Read the model definition and answer for the solid it produces. Units are mm, in the model's axes. Round coordinates to 2 decimals unless told otherwise and drop trailing zeros. Write each loop counter-clockwise with the first axis right and the second up, starting at its lowest first coordinate (ties: lowest second). Pieces come first, ordered by that corner, then holes. Notation, with made-up numbers: (73, 28.25) - (108, 28.25) arc R34 ccw to (108, 66.25) - close; hole circle Ø8 at (-34, 83). An arc over 180 degrees is marked (long way). Use one line per item in the form item = value. Start each with the question number.
1) Each of these flat-tipped pins is pushed along its axis until it touches: pin 1 (1 mm diameter, centred on x = -44, z = 2, fed in from -Y); pin 2 (1.6 mm diameter, centred on x = -27.5, z = 1.5, fed in from -Y); pin 3 (1 mm diameter, centred on y = -2, z = 1, fed in from -X) (3 decimals). Where does it stop, or does it pass through?
2) The part is cut by section C-C, the plane x = -27.5. Give the vertices of the cut face in (y, z) (3 decimals).
3) The part is cut by section B-B, the plane z = 1.35. Give the vertices of the cut face in (x, y) (3 decimals), plus the area to 3 significant figures.
4) Consider line 1 along X through (y, z) = (3.5, 0.85) (3 decimals); line 2 along Y through (x, z) = (-24.5, 2.75); line 3 along Y through (x, z) = (0.5, 2.4). Determine where each line is inside the solid, lowest interval first. Write a range as from..to.
5) The part is cut by section D-D, the plane y = 52.5. Give the vertices of the cut face in (x, z) (3 decimals), plus the area to 3 significant figures.
6) The part is cut by section A-A, the plane y = 3.5. Give the vertices of the cut face in (x, z) (3 decimals), plus the area to 3 significant figures.
from build123d import *

# Parameters (mm, degrees)
BOSS_EXTRUDE1_DEPTH = 3.175
KERF_DEPTH          = 3.175


with BuildPart() as part:
    # Sketch1 → Boss-Extrude1 (new body)
    with BuildSketch(Plane.XY):
        Polygon((0, 0), (-6.35, 0), (-6.35, -3.81), (-19.05, -3.81), (-19.05, 0), (-25.4, 0), (-25.4, 18.4658), (-28.575, 18.4658), (-28.575, 0), (-28.575, -3.81), (-41.275, -3.81), (-41.275, 0), (-47.625, 0), (-47.625, 6.35), (-25.4, 63.5), (0, 63.5), (0, 57.15), (3.048, 57.15), (3.048, 38.1), (0, 38.1), (0, 31.75), (3.048, 31.75), (3.048, 12.7), (0, 12.7), align=None)
    extrude(amount=BOSS_EXTRUDE1_DEPTH)

    # Sketch2 → kerf (add, through all)
    with BuildSketch(Plane.XY.offset(3.175)):
        Polygon((-25.4, 0), (-19.05, 0), (-19.05, -3.81), (-6.35, -3.81), (-6.35, 0), (0, 0), (0, 12.7), (3.048, 12.7), (3.048, 31.75), (0, 31.75), (0, 38.1), (3.048, 38.1), (3.048, 57.15), (0, 57.15), (0, 63.5), (-25.4, 63.5), (-47.625, 6.35), (-47.625, 0), (-41.275, 0), (-41.275, -3.81), (-28.575, -3.81), (-28.575, 18.4658), (-25.4, 18.4658), align=None)
    extrude(amount=-KERF_DEPTH)


solid = part.part
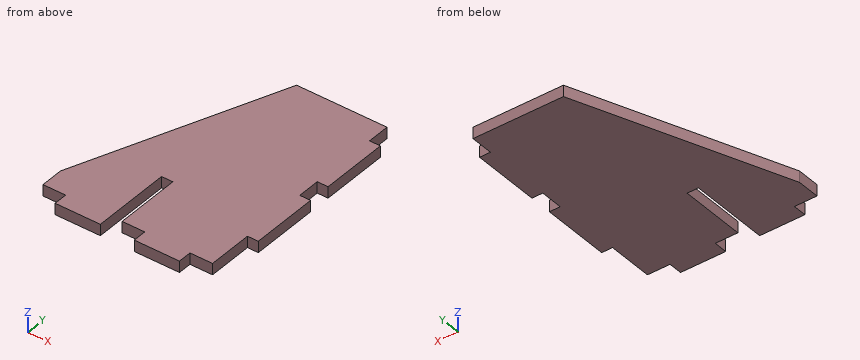
Geometry results:
q1.pin_1 = 0
q1.pin_2 = 18.47
q1.pin_3 = -41.275
q2.outline = (18.466, 0) - (58.1, 0) - (58.1, 3.175) - (18.466, 3.175) - close
q3.outline = (-47.625, 0) - (-41.275, 0) - (-41.275, -3.81) - (-28.575, -3.81) - (-28.575, 18.466) - (-25.4, 18.466) - (-25.4, 0) - (-19.05, 0) - (-19.05, -3.81) - (-6.35, -3.81) - (-6.35, 0) - (0, 0) - (0, 12.7) - (3.048, 12.7) - (3.048, 31.75) - (0, 31.75) - (0, 38.1) - (3.048, 38.1) - (3.048, 57.15) - (0, 57.15) - (0, 63.5) - (-25.4, 63.5) - (-47.625, 6.35) - close
q3.area = 2,540 mm2
q4.line_1 = -47.625..-28.575, -25.4..0
q4.line_2 = 0..63.5
q4.line_3 = 12.7..31.75, 38.1..57.15
q5.outline = (-29.678, 0) - (3.048, 0) - (3.048, 3.175) - (-29.678, 3.175) - close
q5.area = 104 mm2
q6.outline = (-47.625, 0) - (-28.575, 0) - (-28.575, 3.175) - (-47.625, 3.175) - close; (-25.4, 0) - (0, 0) - (0, 3.175) - (-25.4, 3.175) - close
q6.area = 141 mm2
